CAD build for the part. Positions are in the model's coordinates, mm. Face numbers are marked on the shaded views. A direction names the side the tool comes from. Coordinates: 2 decimals unless noted, no trailing zeros. Order: outer loops, then holes, each group sorted by start corner. A loop starts at its lowest first (then second) coordinate and runs counter-clockwise, first axis right, second up. Notation, with made-up numbers: (8.5, 30) - (19.5, 30) arc R3 ccw to (19.5, 34) - close; hole circle Ø3 at (7.25, 27.5). An arc over 180 degrees is marked (long way). Use one line per item in the form item = value.
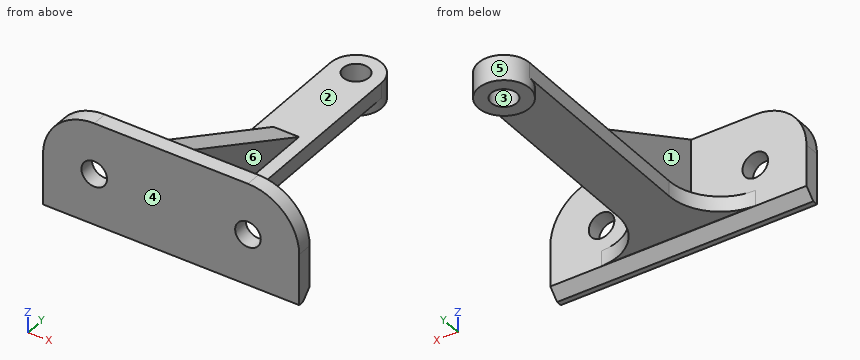
```python
from build123d import *

# Parameters (mm, degrees)
SKETCH1_R           = 6.35
BOSS_EXTRUDE1_DEPTH = 7.62
BOSS_EXTRUDE2_START = -5.08
SKETCH4_R           = 12.7
SKETCH4_R_2         = 6.35
BOSS_EXTRUDE2_DEPTH = 7.62
BOSS_EXTRUDE3_START = 0
SKETCH4_3_R         = 12.7
SKETCH4_3_R_2       = 6.35
BOSS_EXTRUDE3_DEPTH = 5.08
FILLET1_R           = 25.4
RIB1_REACH          = 164.421
SKETCH5_WALL_W      = 412.036258646
SKETCH5_WALL_H      = 12.7
CHAMFER1_SIZE       = 4.92


with BuildPart() as part:
    # Sketch1 → Boss-Extrude1 (new body)
    with BuildSketch(Plane(origin=(0, 0, 0), x_dir=(1, 0, 0), z_dir=(0, 1, 0))):
        with BuildLine():
            Line((-63.5, 25.4), (63.5, 25.4))
            Line((63.5, 25.4), (63.5, 0))
            ThreePointArc((63.5, 0), (56.060512242, -17.960512242), (38.1, -25.4))
            Line((38.1, -25.4), (-38.1, -25.4))
            ThreePointArc((-38.1, -25.4), (-56.060512242, -17.960512242), (-63.5, 0))
            Line((-63.5, 0), (-63.5, 25.4))
        make_face()
        with Locations(Location((-38.1, 0, 0), (0, 0, 90))):
            Circle(SKETCH1_R, mode=Mode.SUBTRACT)
        with Locations(Location((38.1, 0, 0), (0, 0, 90))):
            Circle(SKETCH1_R, mode=Mode.SUBTRACT)
    extrude(amount=BOSS_EXTRUDE1_DEPTH)

    # Sketch4 → Boss-Extrude2 (add)
    # profile 1 of 2: a face of its own
    with BuildSketch(Plane(origin=(0, 0, -25.4), x_dir=(-1, 0, 0), z_dir=(0, 0, -1)).offset(BOSS_EXTRUDE2_START)):
        with BuildLine():
            Line((12.7, 7.62), (12.7, 134.62))
            ThreePointArc((12.7, 134.62), (0, 121.92), (-12.7, 134.62))
            Line((-12.7, 134.62), (-12.7, 7.62))
            Line((-12.7, 7.62), (12.7, 7.62))
        make_face()
    # profile 2 of 2: a face of its own
    with BuildSketch(Plane(origin=(0, 0, -25.4), x_dir=(-1, 0, 0), z_dir=(0, 0, -1)).offset(BOSS_EXTRUDE2_START)):
        with Locations((0, 134.62)):
            Circle(SKETCH4_R)
        with Locations((0, 134.62)):
            Circle(SKETCH4_R_2, mode=Mode.SUBTRACT)
    extrude(amount=-BOSS_EXTRUDE2_DEPTH)

    # Sketch4_3 → Boss-Extrude3 (add)
    with BuildSketch(Plane(origin=(0, 0, -25.4), x_dir=(-1, 0, 0), z_dir=(0, 0, -1)).offset(BOSS_EXTRUDE3_START)):
        with Locations((0, 134.62)):
            Circle(SKETCH4_3_R)
        with Locations((0, 134.62)):
            Circle(SKETCH4_3_R_2, mode=Mode.SUBTRACT)
    extrude(amount=-BOSS_EXTRUDE3_DEPTH)

    # Fillet1
    fillet1_edges = [part.edges().sort_by_distance(p)[0] for p in [
        (-12.7, 7.62, -16.51),
        (12.7, 7.62, -16.51),
    ]]
    fillet(fillet1_edges, radius=FILLET1_R)

    # Sketch5 wall → Rib1 (add, up to next)
    with BuildSketch(Plane(origin=(0, 45.72, 6.35), x_dir=(0, 0.894427191, -0.4472135955), z_dir=(0, 0.4472135955, 0.894427191)), mode=Mode.PRIVATE) as rib1_sk1:
        Rectangle(SKETCH5_WALL_W, SKETCH5_WALL_H)
    rib1_tool1 = extrude(rib1_sk1.sketch, amount=-RIB1_REACH, mode=Mode.PRIVATE) - part.part
    add(rib1_tool1.solids().sort_by_distance((0, 45.72, 6.35))[0])

    # Chamfer1
    chamfer1_edges = [part.edges().sort_by_distance(p)[0] for p in [
        (0, 7.62, -25.4),
    ]]
    chamfer(chamfer1_edges, length=CHAMFER1_SIZE)


solid = part.part
```
Item 1: Cut at B-B, the plane y = 20.5. Write the cut outline in (x, z).
Derived:
outline = (-16, -20.32) - (16, -20.32) - (16, -12.7) - (6.35, -12.7) - (6.35, 18.96) - (-6.35, 18.96) - (-6.35, -12.7) - (-16, -12.7) - close
Item 2: Cut at C-C, the plane z = 15. Write the cut outline in (x, y), plus the area to 3 significant figures.
Derived:
outline = (-58.6, 0) - (58.6, 0) - (58.6, 7.62) - (6.35, 7.62) - (6.35, 28.42) - (-6.35, 28.42) - (-6.35, 7.62) - (-58.6, 7.62) - close
area = 1,160 mm²
Item 3: Drop flat-ended pins along their axis: pin 1 (6 mm diameter, centred on y = 75, z = -15, fed in from +X); pin 2 (3 mm diameter, centred on x = 0.5, y = 44, fed in from -Z); pin 3 (10 mm diameter, centred on x = 38.1, z = 0, fed in from +Y); pin 4 (8.5 mm diameter, centred on y = 75, z = -16.5, fed in from -X). Give the stop position or say it passes through.
Derived:
pin_1 = 12.7
pin_2 = -20.32
pin_3 = through
pin_4 = -12.7
Item 4: Cut at A-A, the plane x = 0. Write the cut outline in (y, z), plus the area to 3 significant figures.
Derived:
outline = (0, -25.4) - (2.7, -25.4) - (7.62, -20.48) - (7.62, -20.32) - (121.92, -20.32) - (121.92, -25.4) - (128.27, -25.4) - (128.27, -12.7) - (83.82, -12.7) - (7.62, 25.4) - (0, 25.4) - close; (140.97, -25.4) - (147.32, -25.4) - (147.32, -12.7) - (140.97, -12.7) - close
area = 2,860 mm²
Item 5: Drill centre lines: line 1 (X direction, y = 4, z = 0); line 2 (Z direction, x = -38.1, y = 2); line 3 (Y direction, x = -43.5, z = 5). Where is each one in solid material? Low to high. Write a range as [from, to].
Derived:
line_1 = [-63.5, -44.45], [-31.75, 31.75], [44.45, 63.5]
line_2 = [-25.4, -6.35], [6.35, 25.4]
line_3 = [0, 7.62]
Item 6: Cut at D-D, the plane x = 46.5. Write the cut outline in (y, z), plus the area to 3 significant figures.
Derived:
outline = (0, -25.4) - (2.7, -25.4) - (7.62, -20.48) - (7.62, 23.97) - (0, 23.97) - close
area = 364 mm²
Item 7: Two-plate mould, pull along Y, no slides. Class the marked faces 4, 5 and 6: +Y half, -Y half, draft (parallel to the pull), parting line (faces both ways), or undercut.
Derived:
face_4 = -Y half
face_5 = undercut
face_6 = draft
Item 8: 3-axis set-ups, long thin cutter, end or side, ignore diameter. For the marked faces 1, 2 and 3: which of +Z, -Z, +X, -X, +Y, -Y reach the whole face in a straight line?
Derived:
face_1 = +Z, -X, +Y
face_2 = +Z, +Y
face_3 = +Z, -Z
